Can you work these out from the model? Positions are in its coordinate system, mm. A direction names the side the tool comes from. Round coordinates to 2 decimals unless told otherwise and drop trailing zeros. Write each loop counter-clockwise with the first axis right and the second up, starting at its lowest first coordinate (ties: lowest second). Pieces come first, ordered by that corner, then holes. Notation, with made-up numbers: (64, 79.25) -> (92, 79.25) arc R11 ccw to (92, 86.25) -> close; hole circle Ø11 at (-38.75, -35). An arc over 180 degrees is marked (long way). Write item = value, one per line. Start each with the question number.
1) Thinking about a two-plate mould opening in X: for faces 4 (the face through (106, -101.922, 19)), 5 (the face through (106, 192.078, 28)), 6 (the face through (349.048, 46, 25)), which applies, +X half, -X half, draft (parallel to the pull), parting line (faces both ways), or undercut?
2) If I drill on line 1 (Y direction, x = 123, z = 7); line 2 (X direction, y = 185.5, z = 14); line 3 (Y direction, x = 115, z = 30.5), over which ranges is the centre line in solid material (lowest first)?
3) Imagine slicing it at A-A, the plane x = -99. Please give me the cut outline in (y, z).
4) I'm going to push flat-ended pins straight in: pin 1 (8 mm diameter, centred on x = -75, z = 12, fed in from -Y); pin 2 (5 mm diameter, centred on x = 121.5, z = 32.5, fed in from -Y); pin 3 (6 mm diameter, centred on x = -54.5, y = 67, fed in from +Z). Where does each tip first touch, or does it pass through?
5) For faces 1 (the face through (115.06, -107.52, 39.42)), 2 (the face through (106, -95.922, 28)), 3 (the face through (106, 50, 0)), which set-ups out of +Z, -Z, +X, -X, +Y, -Y let a thin tool reach every point of the face, with its end or its side?
6) Imagine slicing it at B-B, the plane y = 114.5. Please give me the cut outline in (x, z), then the cut area to 3 significant figures.
from build123d import *

# Parameters (mm, degrees)
F0_W     = 480
F0_H     = 300
F1_DEPTH = 50
F2_T     = -6
F3_R     = 10.1878589924
F4_DEPTH = 20
F4_TAPER = -10
F5_R     = 5


with BuildPart() as f1:
    # F0 (on Top) → F1 (new body)
    with BuildSketch(Plane.XY):
        with Locations((109.0484277904, 48.0776532779)):
            Rectangle(F0_W, F0_H)
    extrude(amount=F1_DEPTH)

    # F2
    f2_openings = [f1.faces().sort_by_distance(p)[0] for p in [
        (109.048428, 48.077653, 50),
    ]]
    offset(amount=F2_T, openings=f2_openings)

    # F3 (on face) → F4 (join)
    with BuildSketch(Plane.XZ.offset(101.9223467221)):
        with Locations((109.0484277904, 30)):
            Circle(F3_R)
    extrude(amount=F4_DEPTH, taper=F4_TAPER)

    # F5
    f5_edges = [f1.edges().sort_by_distance(p)[0] for p in [
        (95.334029, -121.922347, 30),
    ]]
    fillet(f5_edges, radius=F5_R)


solid = f1.part
Reported:
q1.face_4 = draft
q1.face_5 = undercut
q1.face_6 = +X half
q2.line_1 = -101.92 to -95.92, 192.08 to 198.08
q2.line_2 = -130.95 to -124.95, 343.05 to 349.05
q2.line_3 = -121.92 to -95.92, 192.08 to 198.08
q3.outline = (-101.92, 0) -> (198.08, 0) -> (198.08, 50) -> (192.08, 50) -> (192.08, 6) -> (-95.92, 6) -> (-95.92, 50) -> (-101.92, 50) -> close
q4.pin_1 = -101.92
q4.pin_2 = -121.28
q4.pin_3 = 6
q5.face_1 = none
q5.face_2 = +Z
q5.face_3 = -Z, +X, -X, +Y, -Y
q6.outline = (-130.95, 0) -> (349.05, 0) -> (349.05, 50) -> (343.05, 50) -> (343.05, 6) -> (-124.95, 6) -> (-124.95, 50) -> (-130.95, 50) -> close
q6.area = 3,410 mm²
